Design review of the part built by this model. Coordinates are the model's own, in mm. Coordinates: 2 decimals unless noted, no trailing zeros. Loops run counter-clockwise (first coordinate to the right, second up) from the corner with the lowest first, then second, coordinate; pieces in that order, holes last.
from build123d import *

# Parameters (mm, degrees)
ESQUISSE1_R        = 1.5
BOSS_EXTRU_1_DEPTH = 5


with BuildPart() as part:
    # Esquisse1 → Boss.-Extru.1 (new body)
    with BuildSketch(Plane(origin=(0, 0, 0), x_dir=(1, 0, 0), z_dir=(0, 1, 0))):
        with BuildLine():
            Line((-97.415, -97.415), (0, -97.415))
            Line((0, -97.415), (0, -39.915))
            ThreePointArc((0, -39.915), (-28.284271247, -28.199271247), (-40, 0.085))
            Line((-40, 0.085), (-147.415, 0.085))
            Line((-147.415, 0.085), (-147.415, -47.415))
            Line((-147.415, -47.415), (-97.415, -47.415))
            Line((-97.415, -47.415), (-97.415, -97.415))
        make_face()
        with Locations(Location((-12.415, -92.415, 0), (0, 0, 270))):
            Circle(ESQUISSE1_R, mode=Mode.SUBTRACT)
        with Locations(Location((-92.415, -42.415, 0), (0, 0, 270))):
            Circle(ESQUISSE1_R, mode=Mode.SUBTRACT)
        with Locations(Location((-142.415, -12.415, 0), (0, 0, 270))):
            Circle(ESQUISSE1_R, mode=Mode.SUBTRACT)
        with Locations(Location((-31.819805153, -31.734805153, 0), (0, 0, 270))):
            Circle(ESQUISSE1_R, mode=Mode.SUBTRACT)
    extrude(amount=BOSS_EXTRU_1_DEPTH)


solid = part.part
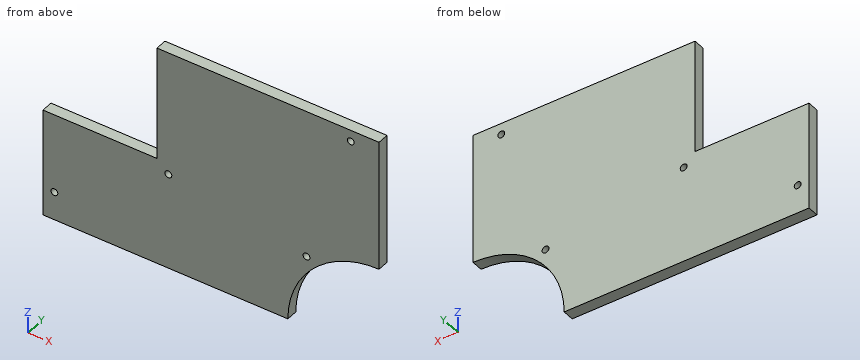
Q1. Take a section at C-C, the plane z = 58.5. Write out the cut boundary in (x, y) (3 decimals), then the cut area to 3 significant figures.
Q2. Take a section at B-B, the plane x = -106.5. Write out the cut boundary in (y, z) (3 decimals).
Q3. For line 1 (Z direction, x = -92.5, y = 4.25) (3 decimals); line 2 (Z direction, x = -106, y = 2.3) (3 decimals); line 3 (X direction, y = 4.05, z = 31) (1 decimal), list the stretches that pass through material, from the lowest coordinate up.
Q4. Clearance check with flat-ended pins moving along their axes: pin 1 Ø2 at (y, z) = (1.5, 22) entering from +X; pin 2 Ø2 at (x, y) = (-28.5, 1) entering from -Z; pin 3 Ø1.5 at (x, y) = (-117.5, 4.5) entering from +Z (3 decimals); pin 4 Ø6 at (x, z) = (-42, 56) entering from -Y. State where each tip first meets the part, or that it passes through.
Q5. Take a section at A-A, the plane y = 1.65. Write out the cut boundary in (x, z) (3 decimals).
Entries:
1. outline: (-97.415, 0) - (0, 0) - (0, 5) - (-97.415, 5) - close
1. area: 487 mm2
2. outline: (0, -0.085) - (5, -0.085) - (5, 47.415) - (0, 47.415) - close
3. line 1: z = -0.085 to 40.917, 43.913 to 97.415
3. line 2: z = -0.085 to 47.415
3. line 3: x = -147.4 to -33.1, -30.5 to -25.2
4. pin 1: stops at x = -32.67
4. pin 2: stops at z = 26.93
4. pin 3: stops at z = 47.415
4. pin 4: stops at y = 0
5. outline: (-147.415, -0.085) - (-40, -0.085) arc R40 cw to (0, 39.915) - (0, 97.415) - (-97.415, 97.415) - (-97.415, 47.415) - (-147.415, 47.415) - close; hole circle Ø3 at (-142.415, 12.415); hole circle Ø3 at (-92.415, 42.415); hole circle Ø3 at (-31.82, 31.735); hole circle Ø3 at (-12.415, 92.415)
